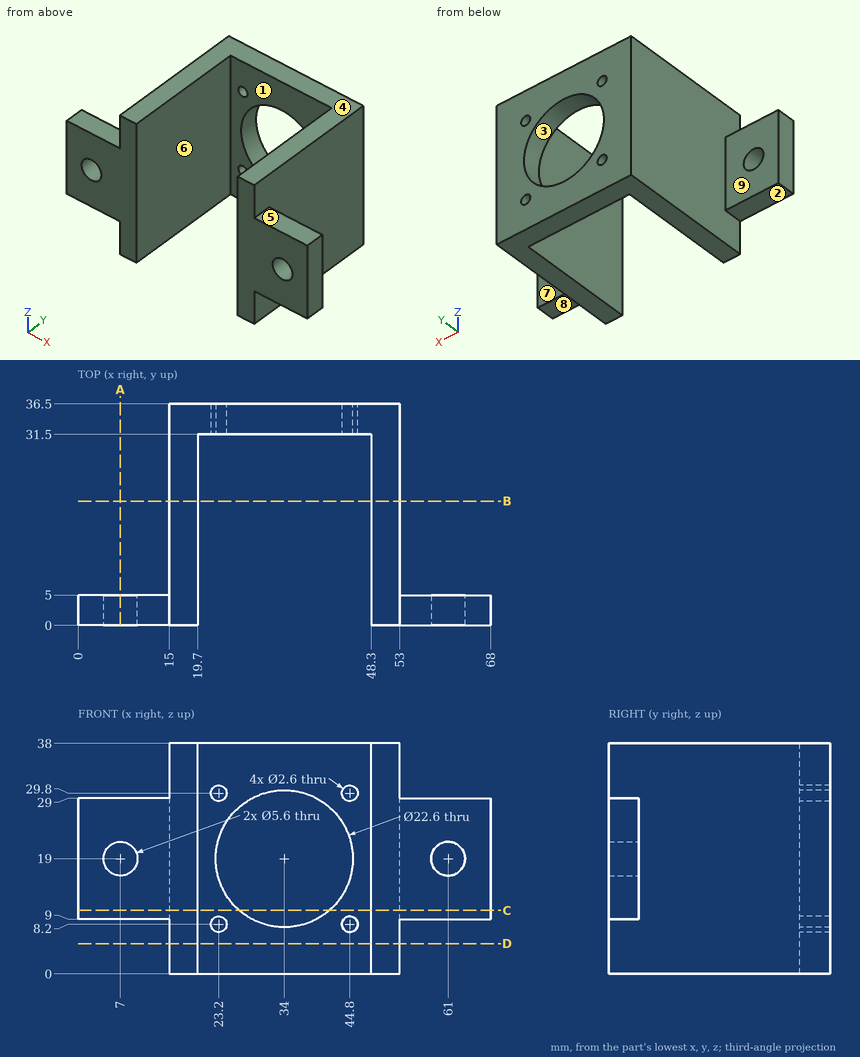
The figure shows three views and two pictorial views of one solid part (mm, origin at its lowest corner). Answer the questions. A direction names the side the tool comes from. Round coordinates to 2 decimals unless told otherwise and drop trailing zeros. Loops run counter-clockwise (first coordinate to the right, second up) from the corner with the lowest first, then second, coordinate; pieces in that order, holes last. Notation, with made-up numbers: (-17.75, 74.5) - (-12.75, 74.5) arc R29 cw to (-12.75, 109.5) - close; hole circle Ø5 at (20, 53). An arc over 180 degrees is marked (long way). One line per question, with ' | ' between items. Start each with the question number.
Q1. Section D-D on z = 5 is taken. Give the vertices of the cut face in (x, y).
Q2. For the marked faces 5, 6, 7, 8 and 9, determine the directions among +Z, -Z, +X, -X, +Y, -Y from which every point of the face is accessible in a straight line to the end or side of a thin tool.
Q3. Section C-C on z = 10.5 is taken. Give the vertices of the cut face in (x, y), plus the area to 3 significant figures.
Q4. For a pull along Z with two mould halves and no side action, classify the marked faces 1, 2, 3 and 4 as +Z half, -Z half, draft (parallel to the pull), parting line (faces both ways), or undercut.
Q5. Section B-B on y = 20.5 is taken. Give the vertices of the cut face in (x, z).
Q6. Section A-A on x = 7 is taken. Give the vertices of the cut face in (y, z).
Q7. Find the intervals of material crossed by L1, parallel to X at y = 8, z = 8; L2, parallel to X at y = 32, z = 29; L3, parallel to Z at x = 7, y = 3, in increasing order.
Q8. Flat-ended cylindrical pins translate along their axes: pin 1 (14.5 mm diameter, centred on x = 37.5, z = 19.5, fed in from -Y); pin 2 (5.5 mm diameter, centred on x = 9.5, y = 3, fed in from +Z); pin 3 (11 mm diameter, centred on y = 24, z = 26, fed in from +X); pin 4 (7.5 mm diameter, centred on x = 61.5, z = 22, fed in from +Y). Find the tip coordinate at first contact, or state that the pin passes through.
Established:
1) outline: (15, 0) - (19.7, 0) - (19.7, 31.5) - (48.3, 31.5) - (48.3, 0) - (53, 0) - (53, 36.5) - (15, 36.5) - close
2) face 5: +Z, +X, +Y, -Y | face 6: +Z, -Z, -Y | face 7: +Z, -Z, +X, +Y | face 8: -Z, +X, +Y, -Y | face 9: +Z, -Z, -X, +Y
3) outline: (0, 0) - (19.7, 0) - (19.7, 31.5) - (26.55, 31.5) - (26.55, 36.5) - (15, 36.5) - (15, 5) - (0, 5) - close; (41.45, 31.5) - (48.3, 31.5) - (48.3, 0) - (68, 0) - (68, 5) - (53, 5) - (53, 36.5) - (41.45, 36.5) - close | area: 562 mm²
4) face 1: draft | face 2: -Z half | face 3: undercut | face 4: +Z half
5) outline: (15, 0) - (19.7, 0) - (19.7, 38) - (15, 38) - close; (48.3, 0) - (53, 0) - (53, 38) - (48.3, 38) - close
6) outline: (0, 9) - (5, 9) - (5, 16.2) - (0, 16.2) - close; (0, 21.8) - (5, 21.8) - (5, 29) - (0, 29) - close
7) L1: 15 to 19.7, 48.3 to 53 | L2: 15 to 22.18, 24.22 to 28.74, 39.26 to 43.78, 45.82 to 53 | L3: 9 to 16.2, 21.8 to 29
8) pin 1: through | pin 2: z = 29 | pin 3: x = 53 | pin 4: y = 5
